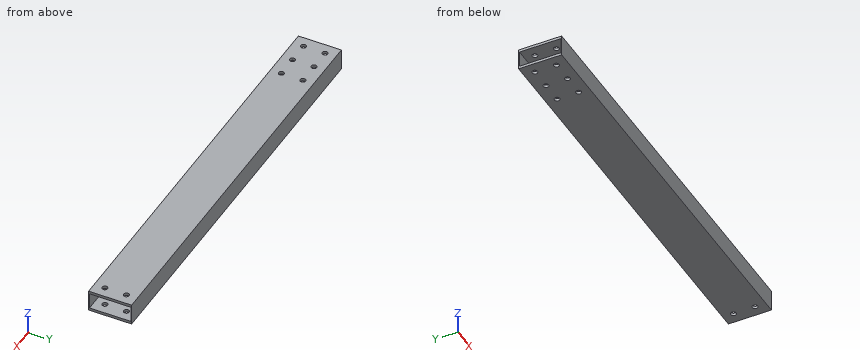
from build123d import *

# Parameters (mm, degrees)
SKETCH1_W               = 25.4
SKETCH1_H               = 50.8
BOSS_EXTRUDE1_DEPTH     = 479.336862
SKETCH2_W               = 19.05
SKETCH2_H               = 48.768
CUT_EXTRUDE1_DEPTH      = 483.689990855
CUT_EXTRUDE4_DEPTH      = 483.689990855
CUT_EXTRUDE4_DEPTH_BACK = 483.689990855
SKETCH5_R               = 3.175


with BuildPart() as part:
    # Sketch1 → Boss-Extrude1 (new body)
    with BuildSketch(Plane(origin=(0, 0, 0), x_dir=(0, 0, -1), z_dir=(1, 0, 0))):
        with Locations((12.7, 25.4)):
            Rectangle(SKETCH1_W, SKETCH1_H)
    extrude(amount=BOSS_EXTRUDE1_DEPTH)

    # Sketch2 → Cut-Extrude1 (cut, through all)
    with BuildSketch(Plane(origin=(479.336862, 0, 0), x_dir=(0, 0, -1), z_dir=(1, 0, 0))):
        with Locations((12.7, 25.4)):
            Rectangle(SKETCH2_W, SKETCH2_H)
    extrude(amount=-CUT_EXTRUDE1_DEPTH, mode=Mode.SUBTRACT)

    # Sketch5 → Cut-Extrude4 (cut, two sides: drawn at the far end of the back side and taken through both)
    with BuildSketch(Plane.XY.offset(-CUT_EXTRUDE4_DEPTH_BACK)):
        with Locations((12.7, 38.1)):
            Circle(SKETCH5_R)
        with Locations((38.1, 38.1)):
            Circle(SKETCH5_R)
        with Locations((12.7, 12.7)):
            Circle(SKETCH5_R)
        with Locations((38.1, 12.7)):
            Circle(SKETCH5_R)
        with Locations((63.5, 38.1)):
            Circle(SKETCH5_R)
        with Locations((63.5, 12.7)):
            Circle(SKETCH5_R)
        with Locations((466.636862, 38.1)):
            Circle(SKETCH5_R)
        with Locations((466.636862, 12.7)):
            Circle(SKETCH5_R)
    extrude(amount=CUT_EXTRUDE4_DEPTH + CUT_EXTRUDE4_DEPTH_BACK, mode=Mode.SUBTRACT)


solid = part.part
Part model, mm, in its own coordinate system. Coordinates: 2 decimals unless noted, no trailing zeros. Order: outer loops, then holes, each group sorted by start corner. A loop starts at its lowest first (then second) coordinate and runs counter-clockwise, first axis right, second up.
(1) Pin check, flat tip, straight feed: pin 1 Ø7.5 at (x, y) = (38.1, 38.1) entering from -Z. Stop position of the tip, or through.
Check sheet entries:
pin 1: stops at z = -25.4
(2) Probe L1, parallel to X at y = 38.1, z = -24.7 (3 decimals); L2, parallel to Y at x = 38.1, z = -24.1 (3 decimals); L3, parallel to Y at x = 337, z = -21.75. List the from-to ranges inside material, lowest first.
Check sheet entries:
L1: x = 0 to 9.525, 15.875 to 34.925, 41.275 to 60.325, 66.675 to 463.462, 469.812 to 479.337
L2: y = 0 to 9.525, 15.875 to 34.925, 41.275 to 50.8
L3: y = 0 to 1.02, 49.78 to 50.8
(3) Slice it at A-A, the plane z = -13. Write the cut outline in (x, y), and give its area (3 significant figures).
Check sheet entries:
outline: (0, 0) - (479.34, 0) - (479.34, 1.02) - (0, 1.02) - close; (0, 49.78) - (479.34, 49.78) - (479.34, 50.8) - (0, 50.8) - close
area: 974 mm2
(4) Slice it at B-B, the plane x = 328. Write the cut outline in (y, z) (3 decimals).
Check sheet entries:
outline: (0, -25.4) - (50.8, -25.4) - (50.8, 0) - (0, 0) - close; hole (1.016, -22.225) - (49.784, -22.225) - (49.784, -3.175) - (1.016, -3.175) - close
